Study the drawing (mm; zero at the part's minimum x, y, z) and answer. A direction names the side the tool comes from. Round coordinates to 2 decimals unless told otherwise and drop trailing zeros. Order: outer loops, then holes, each group sorted by start corner. A loop starts at its lowest first (then second) coordinate and runs counter-clockwise, first axis right, second up. Notation, with made-up numbers: M 78,22.25 L 129,22.25 A15 cw 129,48.25 Z; hole C 63,4.25 d10. An arc over 180 degrees is marked long. Put each result on its own line as item: value. Start each with the question number.
1. The part is cut by section B-B (z = 62.5). Give the vertices of the cut face in (x, y).
2. Consider line 1 (Z direction, x = 2.5, y = 9.25); line 2 (X direction, y = 7, z = 2.5); line 3 (Z direction, x = 3, y = 11). Determine where each line is inside the solid, lowest interval first.
3. The part is cut by section C-C (y = 9). Give the vertices of the cut face in (x, z), then the cut area to 3 significant figures.
4. The part is cut by section D-D (z = 26). Give the vertices of the cut face in (x, y).
5. The part is cut by section A-A (x = 61.5). Give the vertices of the cut face in (y, z), then the cut area to 3 significant figures.
6. Which of the six approach directions +Z, -Z, +X, -X, +Y, -Y give full straight-line access (tool end or side, diameter ignored) to the marked faces 1 and 2?
7. Each of these flat-tipped pins is pushed along its axis until it touches: pin 1 Ø0.8 at (x, y) = (67, 5) entering from +Z; pin 2 Ø1.8 at (x, y) = (67, 5) entering from -Z; pin 3 Ø8 at (x, z) = (18, 51.5) entering from -Y; pin 4 Ø1.9 at (x, z) = (2.5, 62.5) entering from -Y. Where does it stop, or does it pass through?
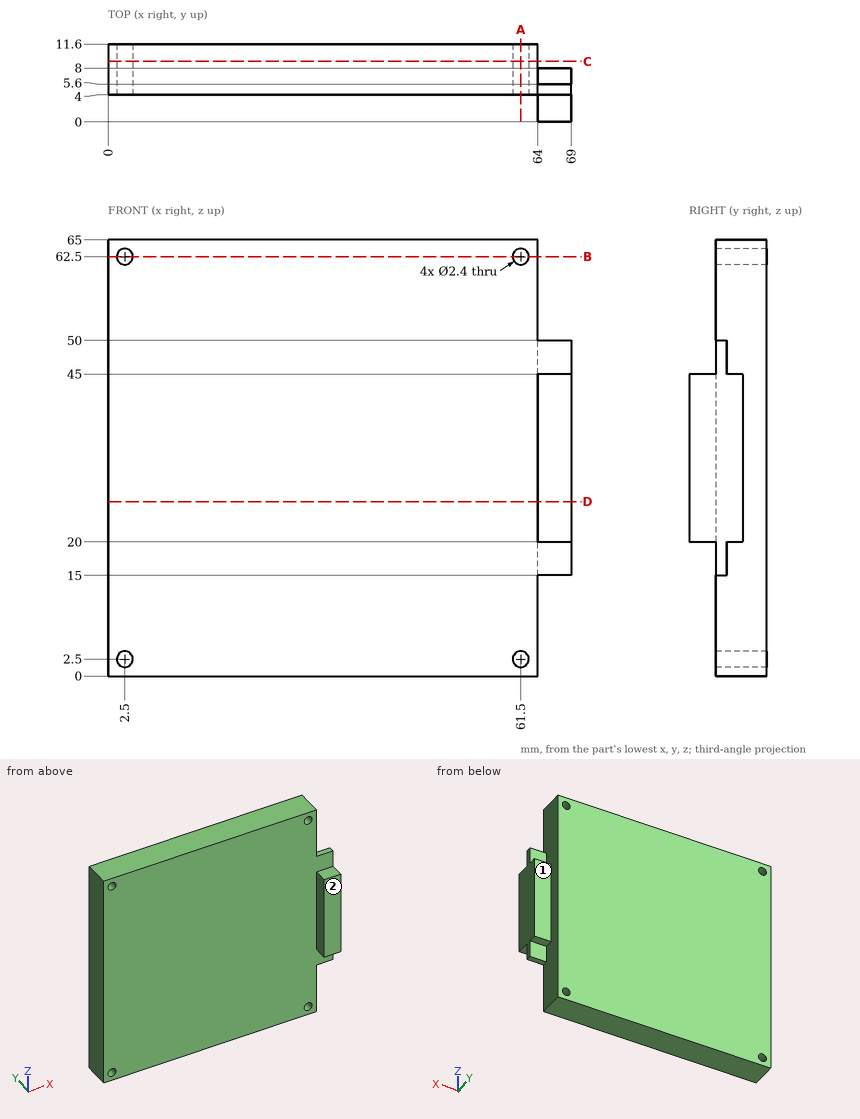
Resolved:
1. outline: M 0,4 L 1.3,4 L 1.3,11.6 L 0,11.6 Z; M 3.7,4 L 60.3,4 L 60.3,11.6 L 3.7,11.6 Z; M 62.7,4 L 64,4 L 64,11.6 L 62.7,11.6 Z
2. line 1: 0 to 1.3, 3.7 to 61.3, 63.7 to 65
2. line 2: 0 to 1.3, 3.7 to 60.3, 62.7 to 64
2. line 3: 0 to 1.41, 3.59 to 61.41, 63.59 to 65
3. outline: M 0,0 L 64,0 L 64,65 L 0,65 Z; hole C 2.5,2.5 d2.4; hole C 2.5,62.5 d2.4; hole C 61.5,2.5 d2.4; hole C 61.5,62.5 d2.4
3. area: 4,140 mm2
4. outline: M 0,4 L 64,4 L 64,0 L 69,0 L 69,8 L 64,8 L 64,11.6 L 0,11.6 Z
5. outline: M 4,0 L 11.6,0 L 11.6,1.3 L 4,1.3 Z; M 4,3.7 L 11.6,3.7 L 11.6,61.3 L 4,61.3 Z; M 4,63.7 L 11.6,63.7 L 11.6,65 L 4,65 Z
5. area: 458 mm2
6. face 1: +Z, -Z, +X, +Y
6. face 2: +Z, -Z, +X, -X, -Y
7. pin 1: z = 50
7. pin 2: z = 15
7. pin 3: y = 4
7. pin 4: through
